from build123d import *
from build123d.topology import SkipClean

# Parameters (mm, degrees)
SKETCH1_R           = 11.1252
SKETCH1_R_2         = 5.588
SKETCH1_R_3         = 1.2065
BOSS_EXTRUDE1_DEPTH = 1.905
BOSS_EXTRUDE2_DEPTH = 9.525
FILLET1_R           = 1.5875


with BuildPart() as part:
    # Sketch1 → Boss-Extrude1 (new body)
    with BuildSketch(Plane(origin=(0, 0, 0), x_dir=(1, 0, 0), z_dir=(0, 1, 0))):
        with Locations(Location((0, 0, 0), (0, 0, 90))):
            Circle(SKETCH1_R)
        with Locations(Location((0, 0, 0), (0, 0, 90))):
            Circle(SKETCH1_R_2, mode=Mode.SUBTRACT)
        with Locations(Location((-7.747, 0, 0), (0, 0, 90))):
            Circle(SKETCH1_R_3, mode=Mode.SUBTRACT)
        with Locations(Location((7.747, 0, 0), (0, 0, 90))):
            Circle(SKETCH1_R_3, mode=Mode.SUBTRACT)
    extrude(amount=BOSS_EXTRUDE1_DEPTH)

    # Sketch2 → Boss-Extrude2 (add)
    with SkipClean():  # the faces are left unmerged after this step: merging them gives an invalid solid
        with BuildSketch(Plane(origin=(0, 1.905, 0), x_dir=(1, 0, 0), z_dir=(0, 1, 0))):
            with BuildLine():
                Line((-9.439954, 1.27), (-11.052474, 1.27))
                ThreePointArc((-11.052474, 1.27), (0, 11.1252), (11.052474, 1.27))
                Line((11.052474, 1.27), (9.439954, 1.27))
                ThreePointArc((9.439954, 1.27), (0, 9.525), (-9.439954, 1.27))
            make_face()
            with BuildLine():
                Line((9.439954, -1.27), (11.052474, -1.27))
                ThreePointArc((11.052474, -1.27), (0, -11.1252), (-11.052474, -1.27))
                Line((-11.052474, -1.27), (-9.439954, -1.27))
                ThreePointArc((-9.439954, -1.27), (0, -9.525), (9.439954, -1.27))
            make_face()
        extrude(amount=BOSS_EXTRUDE2_DEPTH)

    # Fillet1
    fillet1_edges = [part.edges().sort_by_distance(p)[0] for p in [
        (10.246214, 11.43, 1.27),
        (10.246214, 11.43, -1.27),
        (-10.246214, 11.43, -1.27),
        (0, 11.43, -9.525),
        (0, 11.43, 9.525),
        (-10.246214, 11.43, 1.27),
        (9.439954, 6.6675, -1.27),
        (-9.439954, 6.6675, -1.27),
        (-9.439954, 6.6675, 1.27),
        (9.439954, 6.6675, 1.27),
    ]]
    fillet(fillet1_edges, radius=FILLET1_R)


solid = part.part
For this review, take the finished solid that the model builds, in its own axes (mm). A direction names the side the tool comes from. Give positions to 0.01 mm unless a question says otherwise; leave off trailing zeros. Loops run counter-clockwise (first coordinate to the right, second up) from the corner with the lowest first, then second, coordinate; pieces in that order, holes last. Notation, with made-up numbers: M -15,85.5 L 2,85.5 A20 cw 2,107.5 Z; hole C 53,60 d6. An arc over 180 degrees is marked long. Put each result on its own line as item: value. Start each with the question number.
(1) The part is to be moulded in two halves that separate along X. For faces 3 (the flat face through (-3, 0, 5)), 4 (the cylindrical face through (5.455, 0.939, 1.211)), say which applies: +X half, -X half, draft (parallel to the pull), parting line (faces both ways), or undercut.
(2) Machinability: for faces 1 (the cylindrical face through (-8.764, 0.939, -0.649)), 2 (the flat face through (0, 1.905, -6)), which of the approach directions +Z, -Z, +X, -X, +Y, -Y give a long, thin tool a straight path to every point of the face, cutting with its end or side? Answer none if there is none.
(3) For pin 1 (4 mm diameter, centred on x = 5.5, y = 6, fed in from +Z); pin 2 (6 mm diameter, centred on x = 4.5, y = 5.5, fed in from +Z); pin 3 (3 mm diameter, centred on x = -8, y = 6, fed in from -Z), all flat-tipped, find the tip position at first contact; note any pin that passes through.
(4) Add section B-B, the plane z = 0. Write out the cut boundary in (x, y) (1 decimal), then the cut area to 3 significant figures.
(5) Wall thickness on L1, parallel to Z at x = 0.25, y = 6.75; L2, parallel to X at y = 0.45, z = 0; L3, parallel to X at y = 0.5, z = 0.5: over which ranges is each line inside the solid? List them lowest first.
Result:
1. face 3: draft
1. face 4: undercut
2. face 1: +Y, -Y
2. face 2: +Y
3. pin 1: stops at z = 10.56
3. pin 2: stops at z = 11.02
3. pin 3: stops at z = -9.03
4. outline: M -11.1,0 L -9,0 L -9,1.9 L -11.1,1.9 Z; M -6.5,0 L -5.6,0 L -5.6,1.9 L -6.5,1.9 Z; M 5.6,0 L 6.5,0 L 6.5,1.9 L 5.6,1.9 Z; M 9,0 L 11.1,0 L 11.1,1.9 L 9,1.9 Z
4. area: 11.9 mm^2
5. L1: z = -11.12 to -9.52, 9.52 to 11.12
5. L2: x = -11.13 to -8.95, -6.54 to -5.59, 5.59 to 6.54, 8.95 to 11.13
5. L3: x = -11.11 to -8.85, -6.65 to -5.57, 5.57 to 6.65, 8.85 to 11.11
